Geometry check sheet. Reference: the model listing, model coordinates, mm. Face numbers are marked on the shaded views. A direction names the side the tool comes from. Round coordinates to 2 decimals unless told otherwise and drop trailing zeros. Write each loop counter-clockwise with the first axis right and the second up, starting at its lowest first coordinate (ties: lowest second). Pieces come first, ordered by that corner, then holes.
Item 1: Cross-section at D-D (x = -23.5). Enter the section's corners in (y, z).
Item 2: Access from +Z, -Z, +X, -X, +Y, -Y to the whole of each face (thin tool, end or side, straight path). Record for the marked faces 4 and 5.
Item 3: Scan lines: probe 1 along X at (y, z) = (-64.05, -11.5); probe 2 along X at (y, z) = (-62, -11); probe 3 along X at (y, z) = (2.5, 7). Record each from-to range of solid material in increasing order.
Item 4: Draft check along X on the marked faces 1, 2 and 3. Enter one of: pulls with the +X half, pulls with the -X half, needs draft (parallel to the pull), parting line crosses it, or undercut.
Item 5: Cross-section at B-B (z = -17.5). Enter the section's corners in (x, y), then the cut area to 3 significant figures.
Item 6: Cross-section at C-C (y = -61.5). Enter the section's corners in (x, z).
Item 7: Cross-section at A-A (y = 2). State how many separate pieces and enclosed holes the cut face has, then the cut area to 3 significant figures.
Item 8: Depth check by flat-ended pin: P1, Ø1, axis at x = -2.5, z = 24.5, coming from the -Y side; P2, Ø0.9, axis at x = -23, z = 4.5, coming from the +Y side; P3, Ø12, axis at x = -12.5, y = -32, coming from the +Z side; P4, Ø2, axis at x = 29.5, z = -11.5, coming from the -Y side. Enter the tip coordinate at first touch or a pass-through.
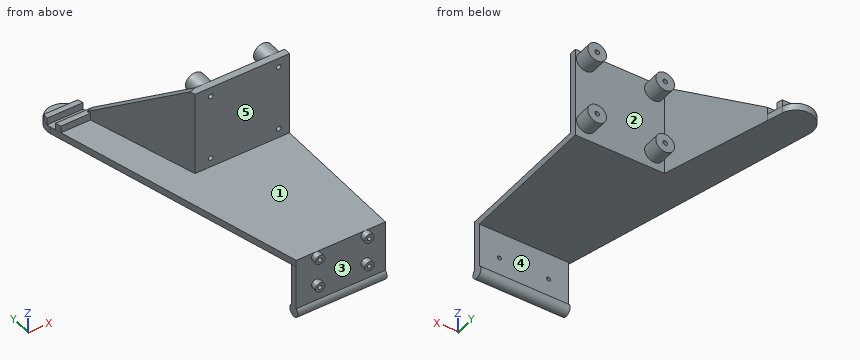
from build123d import *

# Parameters (mm, degrees)
PAD_DEPTH       = 38
SKETCH001_R     = 2.5
PAD001_DEPTH    = 38
SKETCH002_R     = 2
PAD002_DEPTH    = 2.5
SKETCH003_R     = 0.85
POCKET_DEPTH    = 10
SKETCH004_R     = 4
PAD003_DEPTH    = 10
SKETCH005_R     = 1
POCKET001_DEPTH = 10.001
PAD004_DEPTH    = 3
PAD005_DEPTH    = 3
PAD006_DEPTH    = 3
SKETCH009_W     = 60
SKETCH009_H     = 36
POCKET002_DEPTH = 68.001


with BuildPart() as part:
    # Sketch → Pad (new body)
    with BuildSketch(Plane.YZ):
        Polygon((-63, 3), (-63, -23), (-60, -23), (-60, 0), (0, 0), (0, 39), (-3, 39), (-3, 3), align=None)
    extrude(amount=PAD_DEPTH)

    # Sketch001 (on Face10 of Pad) → Pad001 (new body)
    with BuildSketch(Plane.YZ.offset(38)):
        with Locations((-61.5, -21)):
            Circle(SKETCH001_R)
    extrude(amount=-PAD001_DEPTH)

    # Sketch002 (on Face3 of Pad001) → Pad002 (new body)
    with BuildSketch(Plane(origin=(0, -63, 0), x_dir=(0, 0, -1), z_dir=(0, -1, 0))):
        with Locations((-1, 29.5)):
            Circle(SKETCH002_R)
        with Locations((-1, 8.5)):
            Circle(SKETCH002_R)
        with Locations((11.5, 8.5)):
            Circle(SKETCH002_R)
        with Locations((11.5, 29.5)):
            Circle(SKETCH002_R)
    extrude(amount=PAD002_DEPTH)

    # Sketch003 (on Face25 of Pad002) → Pocket (cut)
    with BuildSketch(Plane(origin=(0, -65.5, 0), x_dir=(0, 0, -1), z_dir=(0, -1, 0))):
        with Locations((11.5, 29.5)):
            Circle(SKETCH003_R)
        with Locations((11.5, 8.5)):
            Circle(SKETCH003_R)
        with Locations((-1, 29.5)):
            Circle(SKETCH003_R)
        with Locations((-1, 8.5)):
            Circle(SKETCH003_R)
    extrude(amount=-POCKET_DEPTH, mode=Mode.SUBTRACT)

    # Sketch004 (on Face1 of Pocket) → Pad003 (new body)
    with BuildSketch(Plane(origin=(0, -3, 0), x_dir=(0, 0, -1), z_dir=(0, -1, 0))):
        with Locations((-7, 33.5)):
            Circle(SKETCH004_R)
        with Locations((-7, 4.5)):
            Circle(SKETCH004_R)
        with Locations((-35, 33.5)):
            Circle(SKETCH004_R)
        with Locations((-35, 4.5)):
            Circle(SKETCH004_R)
    extrude(amount=-PAD003_DEPTH)

    # Sketch005 (on Face29 of Pad003) → Pocket001 (cut, through all)
    with BuildSketch(Plane(origin=(0, -3, 0), x_dir=(0, 0, -1), z_dir=(0, -1, 0))):
        with Locations((-35, 33.5)):
            Circle(SKETCH005_R)
        with Locations((-7, 33.5)):
            Circle(SKETCH005_R)
        with Locations((-7, 4.5)):
            Circle(SKETCH005_R)
        with Locations((-35, 4.5)):
            Circle(SKETCH005_R)
    extrude(amount=-POCKET001_DEPTH, mode=Mode.SUBTRACT)

    # Sketch006 (on Face5 of Pocket001) → Pad004 (new body)
    with BuildSketch(Plane.YX):
        with BuildLine():
            Line((0, 0), (51.151245, -15.315145))
            ThreePointArc((47.04327, -29.740249), (56.213208, -24.554175), (51.151245, -15.315145))
            Line((-63, 0), (47.04327, -29.740249))
            Line((-63, 0), (0, 0))
        make_face()
    extrude(amount=-PAD004_DEPTH)

    # Sketch007 (on Face28 of Pad004) → Pad005 (new body)
    with BuildSketch(Plane(origin=(0, 0, 3), x_dir=(0, -1, 0), z_dir=(0, 0, 1))):
        with BuildLine():
            Line((-51.151245, -15.315145), (-48.756291, -14.598074))
            Line((-48.756291, -14.598074), (-48.756291, -29.996039))
            ThreePointArc((-51.151245, -29.684855), (-49.966376, -29.937481), (-48.756291, -29.996039))
            Line((-51.151245, -29.684855), (-51.151245, -15.315145))
        make_face()
        Polygon((-44.756291, -13.400438), (-42.361336, -12.683367), (-42.361336, -28.474911), (-44.756291, -29.122171), align=None)
    extrude(amount=PAD005_DEPTH)

    # Sketch008 (on Face38 of Pad005) → Pad006 (new body)
    with BuildSketch(Plane(origin=(0, 0, 0), x_dir=(-0.286828, 0.957982, 0), z_dir=(0.957982, 0.286828, 0))):
        Polygon((-2.873946, 0), (46.719346, 0), (46.719346, 6), (0, 39), (-2.873946, 39), align=None)
    extrude(amount=-PAD006_DEPTH)

    # Sketch009 (on Face11 of Pad006) → Pocket002 (cut, through all)
    with BuildSketch(Plane.YZ.offset(38)):
        with Locations((-33, 21)):
            Rectangle(SKETCH009_W, SKETCH009_H)
    extrude(amount=-POCKET002_DEPTH, mode=Mode.SUBTRACT)


solid = part.part
Resolved:
1. outline: (23.95, 0) - (56.43, 0) - (56.43, 3) - (51.15, 3) - (51.15, 6) - (48.76, 6) - (48.76, 3) - (44.76, 3) - (44.76, 6) - (42.36, 6) - (42.36, 3) - (23.95, 3) - close
2. face 4: +X, -X, +Y
2. face 5: +Z, +X, -X, -Y
3. probe 1: x = 6.5 to 7.65, 9.35 to 10.5, 27.5 to 28.65, 30.35 to 31.5
3. probe 2: x = 0 to 7.81, 9.19 to 28.81, 30.19 to 38
3. probe 3: x = -3.88 to -0.75, 0.5 to 3.5, 5.5 to 8.5, 29.5 to 32.5, 34.5 to 37.5
4. face 1: needs draft
4. face 2: undercut
4. face 3: undercut
5. outline: (0, -63) - (38, -63) - (38, -60) - (0, -60) - close
5. area: 114 mm2
6. outline: (-0.41, 0) - (0, 0) - (0, -23.5) - (38, -23.5) - (38, 3) - (-0.41, 3) - close; hole circle Ø1.7 at (8.5, -11.5); hole circle Ø1.7 at (8.5, 1); hole circle Ø1.7 at (29.5, -11.5); hole circle Ø1.7 at (29.5, 1)
7. separate pieces: 5
7. enclosed holes: 4
7. area: 347 mm2
8. P1: stops at y = -3
8. P2: stops at y = 51.15
8. P3: stops at z = 3
8. P4: stops at y = -65.5
